Design review of the part built by this model. Coordinates are the model's own, in mm. A direction names the side the tool comes from. Round coordinates to 2 decimals unless told otherwise and drop trailing zeros. Loops run counter-clockwise (first coordinate to the right, second up) from the corner with the lowest first, then second, coordinate; pieces in that order, holes last. Notation, with made-up numbers: (9.5, 82.5) - (46.5, 82.5) arc R11 cw to (46.5, 88.5) - close; hole circle Ø7 at (12, -26.5). An arc over 180 degrees is marked (long way). One line per question, with ' | ' between items. Start each with the question number.
from build123d import *

# Parameters (mm, degrees)
BOSS_EXTRUDE1_DEPTH = 32.5
SKETCH3_R           = 50
SKETCH3_R_2         = 37.5
BOSS_EXTRUDE2_DEPTH = 50
SKETCH4_R           = 37.5
CUT_EXTRUDE1_DEPTH  = 94


with BuildPart() as part:
    # Sketch1 → Boss-Extrude1 (new body, symmetric)
    with BuildSketch(Plane(origin=(0, 0, 0), x_dir=(1, 0, 0), z_dir=(0, 1, 0))):
        Polygon((-89.489291724, 0), (-44.744645862, -77.5), (44.744645862, -77.5), (89.489291724, 0), (44.744645862, 77.5), (-44.744645862, 77.5), align=None)
    extrude(amount=BOSS_EXTRUDE1_DEPTH, both=True)

    # Sketch2 → Cut-Revolve1 (revolve, cut)
    with BuildSketch(Plane.XY):
        with BuildLine():
            Line((-59.489291724, 32.5), (-57.951385683, 32.5))
            Line((-57.951385683, 32.5), (-79.245811776, 59.780712904))
            Line((-79.245811776, 59.780712904), (-106.219123603, 23.051452734))
            Line((-106.219123603, 23.051452734), (-89.489291724, -3.938998624))
            Line((-89.489291724, -3.938998624), (-89.489291724, 2.5))
            ThreePointArc((-89.489291724, 2.5), (-80.70249516, 23.713203436), (-59.489291724, 32.5))
        make_face()
    revolve(axis=Axis((0, 0, 0), (0, 1, 0)), mode=Mode.SUBTRACT)

    # Sketch3 → Boss-Extrude2 (add)
    with BuildSketch(Plane(origin=(0, 32.5, 0), x_dir=(1, 0, 0), z_dir=(0, 1, 0))):
        Circle(SKETCH3_R)
        Circle(SKETCH3_R_2, mode=Mode.SUBTRACT)
    extrude(amount=BOSS_EXTRUDE2_DEPTH)

    # Sketch4 → Cut-Extrude1 (cut)
    with BuildSketch(Plane(origin=(0, 32.5, 0), x_dir=(1, 0, 0), z_dir=(0, 1, 0))):
        Circle(SKETCH4_R)
    extrude(amount=-CUT_EXTRUDE1_DEPTH, mode=Mode.SUBTRACT)


solid = part.part
1. To check wall thickness, follow line 1 along Z through (x, y) = (0, -13); line 2 along Z through (x, y) = (0, 57.5). State the ranges of each line that lie inside material, in increasing order.
2. The part is to be moulded in two halves that separate along X. For faces 3 (the face through (13, 32.5, 49)), 4 (the face through (-66.8, -2.6, -39.3)), 5 (the face through (67.43, -2.59, -38.21)), say which applies: pulls with the +X half, pulls with the -X half, needs draft (parallel to the pull), parting line crosses it, or undercut.
3. Take a section at A-A, the plane x = 0. Give the boundary of the cut face in (y, z), then the cut area to 3 significant figures.
4. Take a section at B-B, the plane y = -13. Give the boundary of the cut face in (x, z), then the cut area to 3 significant figures.
5. Take a section at C-C, the plane y = 15. Give the boundary of the cut face in (x, z).
6. Machinability: for faces 1 (the face through (39, -32.5, -1)), 2 (the face through (47.69, 57.15, -15.02)), which of the approach directions +Z, -Z, +X, -X, +Y, -Y give a long, thin tool a straight path to every point of the face, cutting with its end or side? Answer none if there is none.
7. Clearance check with flat-ended pins moving along their axes: P1, Ø6, axis at x = -53, y = -1, coming from the +Z side; P2, Ø2, axis at y = 44.5, z = 23.5, coming from the -X side; P3, Ø4, axis at y = 1, z = 3.5, coming from the -X side; P4, Ø12, axis at x = 58.5, y = 70, coming from the +Z side. State where each tip first meets the part, or that it passes through.
8. Take a section at D-D, the plane y = 51. Give the boundary of the cut face in (x, z).
Answer list:
1) line 1: z = -77.5 to -37.5, 37.5 to 77.5 | line 2: z = -50 to -37.5, 37.5 to 50
2) face 3: needs draft | face 4: pulls with the -X half | face 5: pulls with the +X half
3) outline: (-32.5, -77.5) - (26.49, -77.5) arc R30 ccw to (32.5, -59.49) - (32.5, -50) - (82.5, -50) - (82.5, -37.5) - (-32.5, -37.5) - close; (-32.5, 37.5) - (82.5, 37.5) - (82.5, 50) - (32.5, 50) - (32.5, 59.49) arc R30 ccw to (26.49, 77.5) - (-32.5, 77.5) - close | area: 6,380 mm²
4) outline: (-89.49, 0) - (-44.74, -77.5) - (44.74, -77.5) - (89.49, 0) - (44.74, 77.5) - (-44.74, 77.5) - close; hole circle Ø75 at (0, 0) | area: 16,400 mm²
5) outline: (-86.62, -4.97) - (-47.62, -72.53) arc R86.76 ccw to (-39, -77.5) - (39, -77.5) arc R86.76 ccw to (47.62, -72.53) - (86.62, -4.97) arc R86.76 ccw to (86.62, 4.97) - (47.62, 72.53) arc R86.76 ccw to (39, 77.5) - (-39, 77.5) arc R86.76 ccw to (-47.62, 72.53) - (-86.62, 4.97) arc R86.76 ccw to start; hole circle Ø75 at (0, 0)
6) face 1: +Z, -Z, +X, -X, -Y | face 2: +Y
7) P1: stops at z = 68.4 | P2: stops at x = -44.65 | P3: stops at x = -88.62 | P4: passes through
8) outline: circle Ø100 at (0, 0); hole circle Ø75 at (0, 0)
